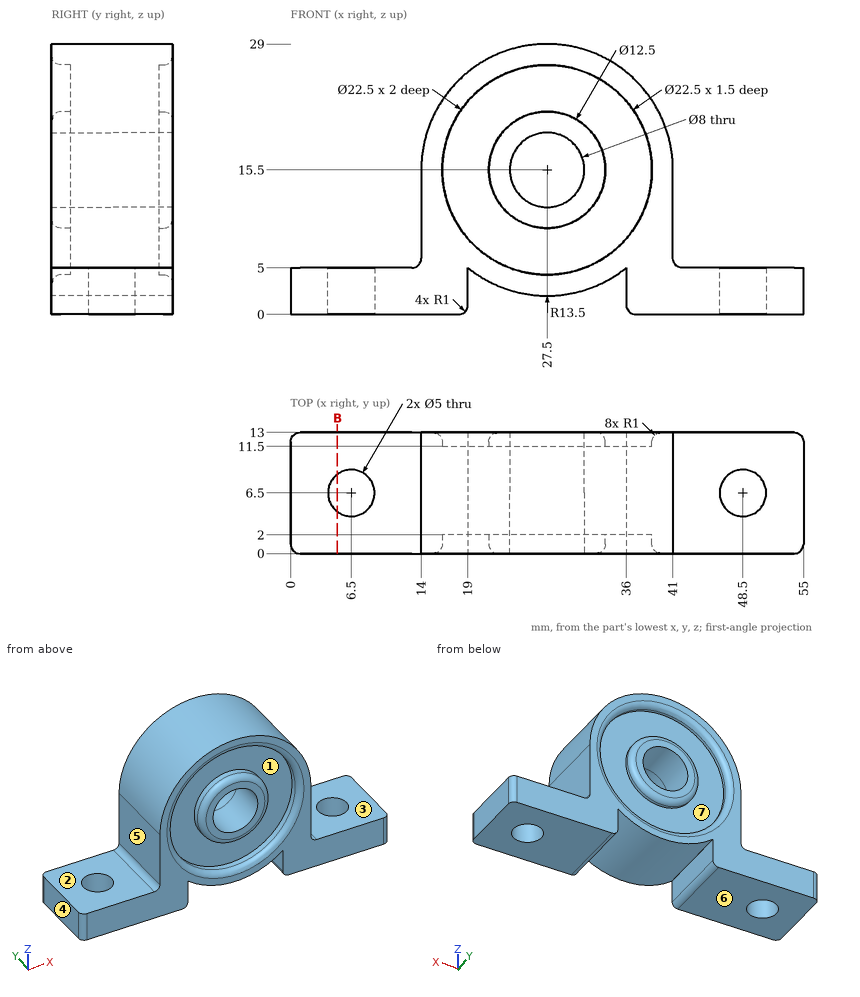
Could you check a few things on this drawing? It's one solid part, dimensions in mm from its lowest x, y, z. A direction names the side the tool comes from. Give positions to 0.01 mm unless a question says otherwise; leave off trailing zeros. Write each loop counter-clockwise with the first axis right and the second up, starting at its lowest first coordinate (ties: lowest second). Pieces come first, ordered by that corner, then holes. Notation, with made-up numbers: (-17.5, 46.5) -> (23.5, 46.5) arc R11 cw to (23.5, 66.5) -> close; hole circle Ø2 at (65, 13). An arc over 180 degrees is marked (long way). Answer as a JSON object with one key per item and string values.
Q1. Please list where these lines run through material, in increasing order: L1, parallel to Y at x = 48.5, z = 2.9; L2, parallel to Z at x = 12.5, y = 9.5; L3, parallel to Y at x = 27, z = 23.75.
Taken from the geometry:
{"L1": "y = 0 to 4, 9 to 13", "L2": "z = 0 to 5", "L3": "y = 2 to 11.5"}
Q2. Which directions (+Z, -Z, +X, -X, +Y, -Y) give clear straight access to the entire face, cutting with the end or side of a thin tool? Please do the marked faces 1, 2, 3 and 4.
Taken from the geometry:
{"face 1": "-Y", "face 2": "+Z, -X, +Y, -Y", "face 3": "+Z, +X, +Y, -Y", "face 4": "+Z, -Z, -X, +Y, -Y"}
Q3. Will these pins go through, and if not, where does the flat tip stop? pin 1 Ø1 at (y, z) = (5, 22.5) entering from -X; pin 2 Ø4 at (x, y) = (9, 6.5) entering from +Z; pin 3 Ø1.5 at (x, y) = (22, 5.5) entering from -Z.
Taken from the geometry:
{"pin 1": "stops at x = 15.67", "pin 2": "stops at z = 5", "pin 3": "stops at z = 2.86"}
Q4. We'd pull the mould along X, two halves only. Please class the marked faces 5, 6 and 7: released by +X, released by -X, zero draft, split by the parting line, or undercut.
Taken from the geometry:
{"face 5": "released by -X", "face 6": "zero draft", "face 7": "undercut"}
Q5. Suppose I cut it at B-B on x = 5. Write out the boundary of the cut face in (y, z), then the cut area to 3 significant figures.
Taken from the geometry:
{"outline": "(0, 0) -> (4.5, 0) -> (4.5, 5) -> (0, 5) -> close; (8.5, 0) -> (13, 0) -> (13, 5) -> (8.5, 5) -> close", "area": "45.0 mm²"}
